Read the model definition and answer for the solid it produces. Units are mm, in the model's axes. Face numbers are marked on the shaded views. A direction names the side the tool comes from. Give positions to 0.01 mm unless a question says otherwise; leave off trailing zeros. Write each loop counter-clockwise with the first axis right and the second up, starting at its lowest first coordinate (ties: lowest second). Pieces come first, ordered by that corner, then holes. Notation, with made-up numbers: (5.25, 26.25) -> (25.25, 26.25) arc R31 cw to (25.25, 55.25) -> close; hole circle Ø11 at (-33, 41). An arc over 180 degrees is marked (long way). Write item = value, one per line.
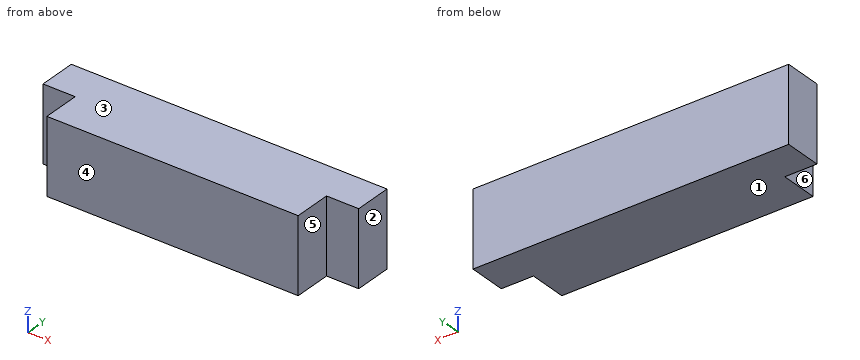
from build123d import *

# Parameters (mm, degrees)
SKETCH1_W           = 42.5
SKETCH1_H           = 6.35
BOSS_EXTRUDE1_DEPTH = 12.7
SKETCH2_W           = 53.3875
SKETCH2_H           = 6.35
BOSS_EXTRUDE2_DEPTH = 12.7


with BuildPart() as part:
    # Sketch1 → Boss-Extrude1 (new body)
    with BuildSketch(Plane.XY):
        Rectangle(SKETCH1_W, SKETCH1_H)
    extrude(amount=BOSS_EXTRUDE1_DEPTH)

    # Sketch2 → Boss-Extrude2 (add)
    with BuildSketch(Plane.XY.offset(12.7)):
        with Locations((0, 6.35)):
            Rectangle(SKETCH2_W, SKETCH2_H)
    extrude(amount=-BOSS_EXTRUDE2_DEPTH)


solid = part.part
(1) The part is cut by section C-C on x = -22. Determine the outline of the cut face in (y, z) (3 decimals), plus the area to 3 significant figures.
Checks:
outline = (3.175, 0) -> (9.525, 0) -> (9.525, 12.7) -> (3.175, 12.7) -> close
area = 80.6 mm²
(2) For a pull along Z with two mould halves and no side action, classify the marked faces 1, 2 and 3 as released by +Z, released by -Z, zero draft, split by the parting line, or undercut.
Checks:
face_1 = released by -Z
face_2 = zero draft
face_3 = released by +Z
(3) The part is cut by section A-A on z = 6.5. Determine the outline of the cut face in (x, y) (3 decimals), plus the area to 3 significant figures.
Checks:
outline = (-26.694, 3.175) -> (-21.25, 3.175) -> (-21.25, -3.175) -> (21.25, -3.175) -> (21.25, 3.175) -> (26.694, 3.175) -> (26.694, 9.525) -> (-26.694, 9.525) -> close
area = 609 mm²
(4) Given P1, Ø3, axis at y = -0.5, z = 4, coming from the +X side; P2, Ø2.5, axis at x = -25, z = 3.5, coming from the -Y side (3 decimals); P3, Ø1.9, axis at y = 1.5, z = 3.5, coming from the -X side, each flat-ended and moving along its own axis, determine where each tip first touches the part or whether it passes through.
Checks:
P1 = 21.25
P2 = 3.175
P3 = -21.25
(5) The part is cut by section B-B on y = 1.75. Determine the outline of the cut face in (x, z).
Checks:
outline = (-21.25, 0) -> (21.25, 0) -> (21.25, 12.7) -> (-21.25, 12.7) -> close
(6) A tool of negligible diameter and unlimited length cuts with its end or side. For the marked faces 4, 5 and 6, from which of +Z, -Z, +X, -X, +Y, -Y can it reach the whole face along a straight path? Write none if from no direction.
Checks:
face_4 = +Z, -Z, +X, -X, -Y
face_5 = +Z, -Z, +X, -Y
face_6 = +Z, -Z, -X, -Y
(7) Consider L1, parallel to X at y = 3, z = 0.75; L2, parallel to Y at x = -23, z = 5 (3 decimals). Determine where each line is inside the solid, lowest interval first.
Checks:
L1 = -21.25 to 21.25
L2 = 3.175 to 9.525
